Build history of the part. All positions in model axes, mm. Give positions to 0.01 mm unless a question says otherwise; leave off trailing zeros. Write each loop counter-clockwise with the first axis right and the second up, starting at its lowest first coordinate (ties: lowest second). Pieces come first, ordered by that corner, then holes. Notation, with made-up numbers: (-34.5, 81) -> (-28.5, 81) arc R11 ccw to (-28.5, 95) -> close; hole circle Ø1 at (75, 54). An arc over 180 degrees is marked (long way). Put each result on its own line as item: value. Start each with the question number.
Item 1: Slice it at A-A, the plane z = 1.75. List the corners of the cut face in (x, y).
Item 2: Slice it at C-C, the plane z = 10.25. List the corners of the cut face in (x, y), plus the area to 3 significant figures.
Item 3: Two-plate mould, pull along Y, no slides. Class faces 1 (the cylindrical face through (18.169, 0.526, 5.824)), 2 (the flat face through (0, 5, 9)), 3 (the flat face through (14.6, -0.1, 0.5)), 4 (the cylindrical face through (-17.89, -1.06, 5.82)): pulls with the +Y half, pulls with the -Y half, needs draft (parallel to the pull), parting line crosses it, or undercut.
Item 4: Slice it at B-B, the plane y = 0. List the corners of the cut face in (x, z), plus the area to 3 significant figures.
Item 5: Drill centre lines: line 1 along Y through (x, z) = (16.5, 8); line 2 along X through (y, z) = (-1.25, 4.5); line 3 along X through (y, z) = (0.75, 9.5). Where is each one in solid material? Low to high.
Item 6: Slice it at D-D, the plane x = 0. List the corners of the cut face in (y, z).
```python
from build123d import *

# Parameters (mm, degrees)
F1_DEPTH = 11
F3_DEPTH = 12.5
F4_R     = 1.75
F5_DEPTH = 25
F6_W     = 45
F6_H     = 1
F7_DEPTH = 12.5


with BuildPart() as f1:
    # F0 (on Top) → F1 (new body)
    with BuildSketch(Plane.XY):
        with BuildLine():
            Line((16.5, 5), (-16.5, 5))
            ThreePointArc((-16.5, 5), (-21.5, 0), (-16.5, -5))
            Line((-16.5, -5), (16.5, -5))
            ThreePointArc((16.5, -5), (21.5, 0), (16.5, 5))
        make_face()
    extrude(amount=F1_DEPTH)

    # F2 (on Front) → F3 (cut, symmetric)
    with BuildSketch(Plane.XZ):
        with BuildLine():
            Line((-8, 0), (8, 0))
            ThreePointArc((8, 0), (0, 8), (-8, 0))
        make_face()
    extrude(amount=F3_DEPTH, both=True, mode=Mode.SUBTRACT)

    # F4 (on face) → F5 (cut)
    with BuildSketch(Plane.XY.offset(11)):
        with Locations((-16.5, 0)):
            Circle(F4_R)
        with Locations((16.5, 0)):
            Circle(F4_R)
    extrude(amount=-F5_DEPTH, mode=Mode.SUBTRACT)

    # F6 (on Front) → F7 (cut, symmetric)
    with BuildSketch(Plane.XZ):
        Rectangle(F6_W, F6_H)
    extrude(amount=F7_DEPTH, both=True, mode=Mode.SUBTRACT)


solid = f1.part
```
Values follow:
1. outline: (-16.5, -5) -> (-7.81, -5) -> (-7.81, 5) -> (-16.5, 5) arc R5 ccw to start; (7.81, -5) -> (16.5, -5) arc R5 ccw to (16.5, 5) -> (7.81, 5) -> close; hole circle Ø3.5 at (-16.5, 0); hole circle Ø3.5 at (16.5, 0)
2. outline: (-16.5, -5) -> (16.5, -5) arc R5 ccw to (16.5, 5) -> (-16.5, 5) arc R5 ccw to start; hole circle Ø3.5 at (-16.5, 0); hole circle Ø3.5 at (16.5, 0)
2. area: 389 mm2
3. face 1: undercut
3. face 2: pulls with the +Y half
3. face 3: needs draft
3. face 4: undercut
4. outline: (-21.5, 0.5) -> (-18.25, 0.5) -> (-18.25, 11) -> (-21.5, 11) -> close; (-14.75, 0.5) -> (-7.98, 0.5) arc R8 cw to (7.98, 0.5) -> (14.75, 0.5) -> (14.75, 11) -> (-14.75, 11) -> close; (18.25, 0.5) -> (21.5, 0.5) -> (21.5, 11) -> (18.25, 11) -> close
4. area: 285 mm2
5. line 1: -5 to -1.75, 1.75 to 5
5. line 2: -21.34 to -17.72, -15.28 to -6.61, 6.61 to 15.28, 17.72 to 21.34
5. line 3: -21.44 to -18.08, -14.92 to 14.92, 18.08 to 21.44
6. outline: (-5, 8) -> (5, 8) -> (5, 11) -> (-5, 11) -> close
